Source: CAD feature listing. Evaluate the final solid. Frame: model axes, mm. Face numbers are marked on the shaded views. A direction names the side the tool comes from. Round coordinates to 2 decimals unless told otherwise and drop trailing zeros. Write each loop counter-clockwise with the first axis right and the second up, starting at its lowest first coordinate (ties: lowest second). Pieces come first, ordered by that corner, then holes. Notation, with made-up numbers: M 17.25,-25.75 L 28.25,-25.75 A30 cw 28.25,10.25 Z; hole C 21.5,27 d6. An arc over 180 degrees is marked long. Answer in a Markdown table with one row per item.
from build123d import *

# Parameters (mm, degrees)
SKETCH_1_W         = 32
SKETCH_1_H         = 32
SKETCH_1_R         = 1.25
EXTRUDE_1472_DEPTH = 1.5
EXTRUDE_START      = 1.5
SKETCH_1_3_W       = 22.3
SKETCH_1_3_H       = 5.5
EXTRUDE_1647_DEPTH = 2.5
SKETCH_1_4_R       = 6.9
SKETCH_1_4_R_2     = 6
EXTRUDE_1817_DEPTH = 8
EXTRUDE_START_2    = 9.5
SKETCH_1_5_R       = 6
EXTRUDE_1989_DEPTH = 3.5
EXTRUDE_START_3    = 13
SKETCH_1_6_R       = 8
SKETCH_1_6_R_2     = 6.9
SKETCH_1_6_R_3     = 6
EXTRUDE_2083_DEPTH = 6
SKETCH_1_7_R       = 1.5
EXTRUDE_2264_DEPTH = 0.5
SKETCH_2_W         = 16
SKETCH_2_H         = 1
EXTRUDE_2724_DEPTH = 10
SKETCH_3_W         = 16
SKETCH_3_H         = 1
EXTRUDE_3021_DEPTH = 10


with BuildPart() as part:
    # Эскиз1 → Extrude 1472 (new body)
    with BuildSketch(Plane.XY):
        Rectangle(SKETCH_1_W, SKETCH_1_H)
        with Locations((-14.25, -14.25)):
            Circle(SKETCH_1_R, mode=Mode.SUBTRACT)
        with Locations((14.25, -14.25)):
            Circle(SKETCH_1_R, mode=Mode.SUBTRACT)
        with Locations((-14.25, 14.25)):
            Circle(SKETCH_1_R, mode=Mode.SUBTRACT)
        with Locations((14.25, 14.25)):
            Circle(SKETCH_1_R, mode=Mode.SUBTRACT)
    extrude(amount=EXTRUDE_1472_DEPTH)

    # Эскиз1<3> → Extrude 1647 (add)
    with BuildSketch(Plane.XY.offset(EXTRUDE_START)):
        with Locations((0, -13.25)):
            Rectangle(SKETCH_1_3_W, SKETCH_1_3_H)
    extrude(amount=EXTRUDE_1647_DEPTH)

    # Эскиз1<4> → Extrude 1817 (add)
    with BuildSketch(Plane.XY.offset(EXTRUDE_START)):
        Circle(SKETCH_1_4_R)
        Circle(SKETCH_1_4_R_2, mode=Mode.SUBTRACT)
        Circle(SKETCH_1_4_R_2)
    extrude(amount=EXTRUDE_1817_DEPTH)

    # Эскиз1<5> → Extrude 1989 (add)
    with BuildSketch(Plane.XY.offset(EXTRUDE_START_2)):
        Circle(SKETCH_1_5_R)
    extrude(amount=EXTRUDE_1989_DEPTH)

    # Эскиз1<6> → Extrude 2083 (add)
    with BuildSketch(Plane.XY.offset(EXTRUDE_START_3)):
        Circle(SKETCH_1_6_R)
        Circle(SKETCH_1_6_R_2, mode=Mode.SUBTRACT)
        Circle(SKETCH_1_6_R_2)
        Circle(SKETCH_1_6_R_3, mode=Mode.SUBTRACT)
        Circle(SKETCH_1_6_R_3)
    extrude(amount=EXTRUDE_2083_DEPTH)

    # Эскиз1<7> → Extrude 2264 (add)
    with BuildSketch(Plane.XY):
        with Locations((9.5, 0)):
            Circle(SKETCH_1_7_R)
        with Locations((-9.5, 0)):
            Circle(SKETCH_1_7_R)
    extrude(amount=-EXTRUDE_2264_DEPTH)

    # Эскиз2 → Extrude 2724 (add)
    with BuildSketch(Plane.XZ.offset(16)):
        with Locations((0, 3)):
            Rectangle(SKETCH_2_W, SKETCH_2_H)
    extrude(amount=EXTRUDE_2724_DEPTH)

    # Эскиз3 → Extrude 3021 (add)
    with BuildSketch(Plane(origin=(0, 0, 2.5), x_dir=(-1, 0, 0), z_dir=(0, 0, -1))):
        with Locations((0, -25.5)):
            Rectangle(SKETCH_3_W, SKETCH_3_H)
    extrude(amount=EXTRUDE_3021_DEPTH)


solid = part.part
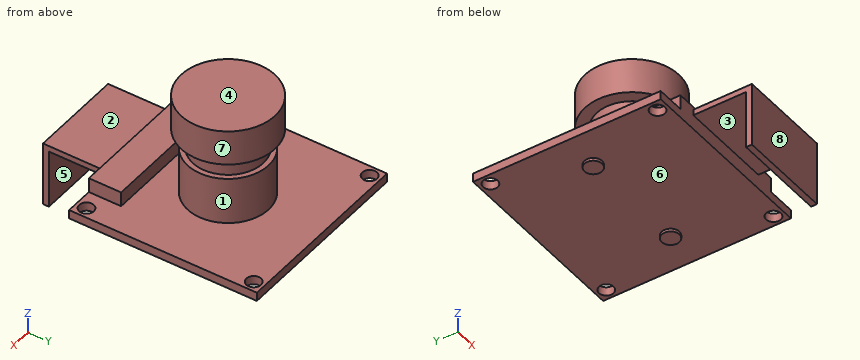
Q1. Access query for the marked faces 1, 2, 3 and 4. Directions: +Z, -Z, +X, -X, +Y, -Y. A direction counts if a zero-diameter tool reaches every point of the face in a straight line with its end or side. Return the directions, or none.
Solutions:
| item | result |
|---|---|
| face 1 | none |
| face 2 | +Z, +X, -X, -Y |
| face 3 | -Z, +X, -X |
| face 4 | +Z, +X, -X, +Y, -Y |
Q2. Section A-A (x = -14.25). Return loops of the section in (y, z).
Solutions:
| item | result |
|---|---|
| outline | M -16,0 L -15.5,0 L -15.5,1.5 L -16,1.5 Z; M -13,0 L 13,0 L 13,1.5 L -13,1.5 Z; M 15.5,0 L 16,0 L 16,1.5 L 15.5,1.5 Z |
Q3. Pull-direction query (Y, two-part tool) for the marked faces 5, 6, 7 and 8; classes: pulls with the +Y half, pulls with the -Y half, needs draft (parallel to the pull), parting line crosses it, or undercut.
Solutions:
| item | result |
|---|---|
| face 5 | undercut |
| face 6 | needs draft |
| face 7 | parting line crosses it |
| face 8 | pulls with the -Y half |
Q4. Section C-C (x = 0). Return loops of the section in (y, z), and give its area (3 significant figures).
Solutions:
| item | result |
|---|---|
| outline | M -26,-7.5 L -25,-7.5 L -25,2.5 L -16,2.5 L -16,0 L 16,0 L 16,1.5 L 6.9,1.5 L 6.9,9.5 L 6,9.5 L 6,13 L 8,13 L 8,19 L -8,19 L -8,13 L -6,13 L -6,9.5 L -6.9,9.5 L -6.9,1.5 L -10.5,1.5 L -10.5,4 L -16,4 L -16,3.5 L -26,3.5 Z |
| area | 330 mm2 |
Q5. Section B-B (y = -14.25). Return loops of the section in (x, z), and give its area (4 significant figures).
Solutions:
| item | result |
|---|---|
| outline | M -16,0 L -15.5,0 L -15.5,1.5 L -16,1.5 Z; M -13,0 L 13,0 L 13,1.5 L 11.15,1.5 L 11.15,4 L -11.15,4 L -11.15,1.5 L -13,1.5 Z; M 15.5,0 L 16,0 L 16,1.5 L 15.5,1.5 Z |
| area | 96.25 mm2 |
Q6. Section D-D (z = 10.25). Return loops of the section in (x, y), and give its area (3 significant figures).
Solutions:
| item | result |
|---|---|
| outline | C 0,0 d12 |
| area | 113 mm2 |
Q7. Contact query for flat-ended pins moving along their axis: pin 1 Ø2 at (y, z) = (-14, 3) entering from +X; pin 2 Ø4 at (y, z) = (7, 12) entering from +X; pin 3 Ø4 at (x, y) = (14.25, -14.25) entering from +Z. Output: stop coordinate, or through.
Solutions:
| item | result |
|---|---|
| pin 1 | stops at x = 11.15 |
| pin 2 | stops at x = 6.02 |
| pin 3 | stops at z = 1.5 |
Q8. Material intervals for probe 1 along Y at (x, z) = (14.25, 0.8); probe 2 along Y at (x, z) = (-0.5, 1.25); probe 3 along Z at (x, y) = (7.5, 1), sorted ascending.
Solutions:
| item | result |
|---|---|
| probe 1 | y = -16 to -15.5, -13 to 13, 15.5 to 16 |
| probe 2 | y = -26 to -25, -16 to 16 |
| probe 3 | z = 0 to 1.5, 13 to 19 |
